Autodesk Inventor part; units mm, degrees
ref_plane "YZ Plane" through (0, 0, 0) normal (1, 0, 0) x (0, 1, 0)
ref_plane "XZ Plane" through (0, 0, 0) normal (0, 1, 0) x (-1, 0, 0)
ref_plane "XY Plane" through (0, 0, 0) normal (0, 0, 1) x (1, 0, 0)
sketch "Sketch1" plane through (0, 0, 0) normal (1, 0, 0) x (0, 1, 0)
  line L0 (0, -1) -> (0, 6)
  line L1 (-2.8, 0) -> (2.8, 0)
  line L2 (-2, 1.44) -> (2, 1.44)
  line L3 (2, 1.44) -> (2, 1.94)
  line L4 (2, 1.94) -> (1.8, 1.94)
  line L5 (1.8, 1.94) -> (1.8, 4.14)
  line L6 (1.8, 4.14) -> (2, 4.5)
  line L7 (2, 4.5) -> (2, 5)
  line L8 (2, 5) -> (-2, 5)
  line L9 (-2, 5) -> (-2, 4.5)
  line L10 (-2, 4.5) -> (-1.8, 4.14)
  line L11 (-1.8, 4.14) -> (-1.8, 1.94)
  line L12 (-1.8, 1.94) -> (-2, 1.94)
  line L13 (-2, 1.94) -> (-2, 1.44)
  point P0 (0, 0)
  dimension "d0" = 2.88
  dimension "d1" = 10
  dimension "d2" = 4
  dimension "d3" = 0.5
  dimension "d4" = 0.5
  dimension "d5" = 2.2
  dimension "d6" = 0.2
revolve "Revolution1" add sketch "Sketch1" angle 360 about axis through (0, -10, 0) along (0, 1, 0)
properties part number "empty"
Model file for the job. Use its own axes, mm. A direction names the side the tool comes from. Coordinates: 2 decimals unless noted, no trailing zeros. Write each loop counter-clockwise with the first axis right and the second up, starting at its lowest first coordinate (ties: lowest second). Pieces come first, ordered by that corner, then holes. Notation, with made-up numbers: (68, -23.5) - (87, -23.5) arc R19 cw to (87, -12.5) - close; hole circle Ø5 at (21, -17.75). An arc over 180 degrees is marked (long way). One line per item, written item: value. Start each with the question number.
1. Slice it at B-B (x = 0). Write the cut outline in (y, z), plus the area to 3 significant figures.
2. Flat gauge pins, fed straight in: pin 1 (2.5 mm diameter, centred on x = 0, z = 0, fed in from +Y); pin 2 (2 mm diameter, centred on x = -3.5, y = -1, fed in from +Z); pin 3 (1 mm diameter, centred on x = -2.5, y = 1.5, fed in from -Z). Where does each tip first touch, or does it go through?
3. Probe line 1 (X direction, y = 0.45, z = 0); line 2 (Y direction, x = -2.5, z = 2.5); line 3 (X direction, y = 0.3, z = -2.25). List the from-to ranges inside material, lowest first. Write a range as from..to.
4. Slice it at A-A (z = 0). Write the cut outline in (x, y), plus the area to 3 significant figures.
5. Slice it at C-C (y = 1.35). Write the cut outline in (x, z), plus the area to 3 significant figures.
6. Mould opens along X. For faces 1 (the cylindrical face through (4.88, -0.03, -1.08)), 2 (the flat face through (-1, -1.8, 2)) say: released by +X, released by -X, zero draft, split by the parting line, or undercut.
7. Tool access for faces 3 (the cylindrical face through (0.433, 0.028, 1.374)), 4 (the flat face through (-1, 1.8, 2)): list every direction of +Z, -Z, +X, -X, +Y, -Y with a clear straight run to the whole face (end or side of a thin tool).
Answers below:
1. outline: (-2, -5) - (2, -5) - (2, -4.5) - (1.8, -4.14) - (1.8, -1.94) - (2, -1.94) - (2, -1.44) - (-2, -1.44) - (-2, -1.94) - (-1.8, -1.94) - (-1.8, -4.14) - (-2, -4.5) - close; (-2, 1.44) - (2, 1.44) - (2, 1.94) - (1.8, 1.94) - (1.8, 4.14) - (2, 4.5) - (2, 5) - (-2, 5) - (-2, 4.5) - (-1.8, 4.14) - (-1.8, 1.94) - (-2, 1.94) - close
1. area: 26.6 mm^2
2. pin 1: passes through
2. pin 2: stops at z = 4.33
2. pin 3: stops at z = -4.58
3. line 1: x = -5..-1.44, 1.44..5
3. line 2: y = -1.8..1.8
3. line 3: x = -4.47..4.47
4. outline: (-5, -2) - (-4.5, -2) - (-4.14, -1.8) - (-1.94, -1.8) - (-1.94, -2) - (-1.44, -2) - (-1.44, 2) - (-1.94, 2) - (-1.94, 1.8) - (-4.14, 1.8) - (-4.5, 2) - (-5, 2) - close; (1.44, -2) - (1.94, -2) - (1.94, -1.8) - (4.14, -1.8) - (4.5, -2) - (5, -2) - (5, 2) - (4.5, 2) - (4.14, 1.8) - (1.94, 1.8) - (1.94, 2) - (1.44, 2) - close
4. area: 26.6 mm^2
5. outline: circle Ø10 at (0, 0); hole circle Ø2.88 at (0, 0)
5. area: 72.0 mm^2
6. face 1: split by the parting line
6. face 2: undercut
7. face 3: +Y, -Y
7. face 4: +Y
